Read the model definition and answer for the solid it produces. Units are mm, in the model's axes. A direction names the side the tool comes from. Give positions to 0.01 mm unless a question says otherwise; leave off trailing zeros. Loops run counter-clockwise (first coordinate to the right, second up) from the corner with the lowest first, then second, coordinate; pieces in that order, holes last. Notation, with made-up numbers: (80.5, -39) - (123.5, -39) arc R16 cw to (123.5, -27) - close; hole circle Ø3 at (0.25, 13). An arc over 180 degrees is marked (long way). Put each result on its own line as item: value. Start each with the question number.
1. Consider L1, parallel to Z at x = 24.95, y = 13.2; L2, parallel to X at y = 7.5, z = 6.75. Determine where each line is inside the solid, lowest interval first. Write a range as from..to.
2. For faces 1 (the flat face through (13, 13, 6)), 2 (the cylindrical face through (0.57, 0.6, 11.15)), determine the directions among +Z, -Z, +X, -X, +Y, -Y from which every point of the face is accessible in a straight line to the end or side of a thin tool.
3. For a pull along Z with two mould halves and no side action, classify faces 3 (the flat face through (13, 13, 0)), 4 (the cylindrical face through (24.92, 12.83, 13.34)), 5 (the flat face through (26.4, 13, 11)) as released by +Z, released by -Z, zero draft, split by the parting line, or undercut.
4. A cutting plane is placed at A-A, the plane z = 15. Determine the outline of the cut face in (x, y).
5. A cutting plane is placed at B-B, the plane y = 13.2. Determine the outline of the cut face in (x, z).
6. Given pin 1 Ø3 at (x, y) = (19, 9.5) entering from +Z, flat-ended and moving along its own axis, determine where the tip first touches the part or whether it passes through.
7. A cutting plane is placed at C-C, the plane x = 15.5. Determine the outline of the cut face in (y, z), plus the area to 3 significant figures.
8. A cutting plane is placed at D-D, the plane z = 19.25. Determine the outline of the cut face in (x, y), plus the area to 3 significant figures.
```python
from build123d import *

# Parameters (mm, degrees)
BOX_W           = 26.4
BOX_H           = 26.4
BOX_DEPTH       = 22
SKETCH_W        = 20.4
SKETCH_H        = 20.4
POCKET_DEPTH    = 16
FILLET_R        = 2
SKETCH001_R     = 1.7
POCKET001_DEPTH = 5


with BuildPart() as part:
    # Box → Box (new body)
    with BuildSketch(Plane.XY):
        with Locations((13.2, 13.2)):
            Rectangle(BOX_W, BOX_H)
    extrude(amount=BOX_DEPTH)

    # Sketch → Pocket (cut)
    with BuildSketch(Plane.XY.offset(22)):
        with Locations((13.2, 13.2)):
            Rectangle(SKETCH_W, SKETCH_H)
    extrude(amount=-POCKET_DEPTH, mode=Mode.SUBTRACT)

    # Fillet
    fillet_edges = [part.edges().sort_by_distance(p)[0] for p in [
        (0, 26.4, 11),
        (26.4, 26.4, 11),
        (26.4, 0, 11),
        (0, 0, 11),
    ]]
    fillet(fillet_edges, radius=FILLET_R)

    # Sketch001 → Pocket001 (cut)
    with BuildSketch(Plane.YZ.offset(26.4)):
        with Locations((13.2, 15)):
            Circle(SKETCH001_R)
    extrude(amount=-POCKET001_DEPTH, mode=Mode.SUBTRACT)


solid = part.part
```
Return value:
1. L1: z = 0..13.3, 16.7..22
1. L2: x = 0..3, 23.4..26.4
2. face 1: +Z
2. face 2: +Z, -Z, -X, -Y
3. face 3: released by -Z
3. face 4: undercut
3. face 5: zero draft
4. outline: (0, 2) arc R2 ccw to (2, 0) - (24.4, 0) arc R2 ccw to (26.4, 2) - (26.4, 11.5) - (23.4, 11.5) - (23.4, 3) - (3, 3) - (3, 23.4) - (23.4, 23.4) - (23.4, 14.9) - (26.4, 14.9) - (26.4, 24.4) arc R2 ccw to (24.4, 26.4) - (2, 26.4) arc R2 ccw to (0, 24.4) - close
5. outline: (0, 0) - (26.4, 0) - (26.4, 13.3) - (23.4, 13.3) - (23.4, 6) - (3, 6) - (3, 22) - (0, 22) - close; (23.4, 16.7) - (26.4, 16.7) - (26.4, 22) - (23.4, 22) - close
6. pin 1: stops at z = 6
7. outline: (0, 0) - (26.4, 0) - (26.4, 22) - (23.4, 22) - (23.4, 6) - (3, 6) - (3, 22) - (0, 22) - close
7. area: 254 mm2
8. outline: (0, 2) arc R2 ccw to (2, 0) - (24.4, 0) arc R2 ccw to (26.4, 2) - (26.4, 24.4) arc R2 ccw to (24.4, 26.4) - (2, 26.4) arc R2 ccw to (0, 24.4) - close; hole (3, 3) - (23.4, 3) - (23.4, 23.4) - (3, 23.4) - close
8. area: 277 mm2
